Study the drawing (mm; zero at the part's minimum x, y, z) and answer. A direction names the side the tool comes from. Round coordinates to 2 decimals unless told otherwise and drop trailing zeros. Write each loop counter-clockwise with the first axis right and the second up, starting at its lowest first coordinate (ties: lowest second). Pieces come first, ordered by that corner, then holes. Notation, with made-up numbers: M 1,34 L 33,34 A23 cw 33,62 Z; hole C 45,-40 d10. An arc over 180 degrees is marked long. Write each question's results on one line, items separated by ' | '.
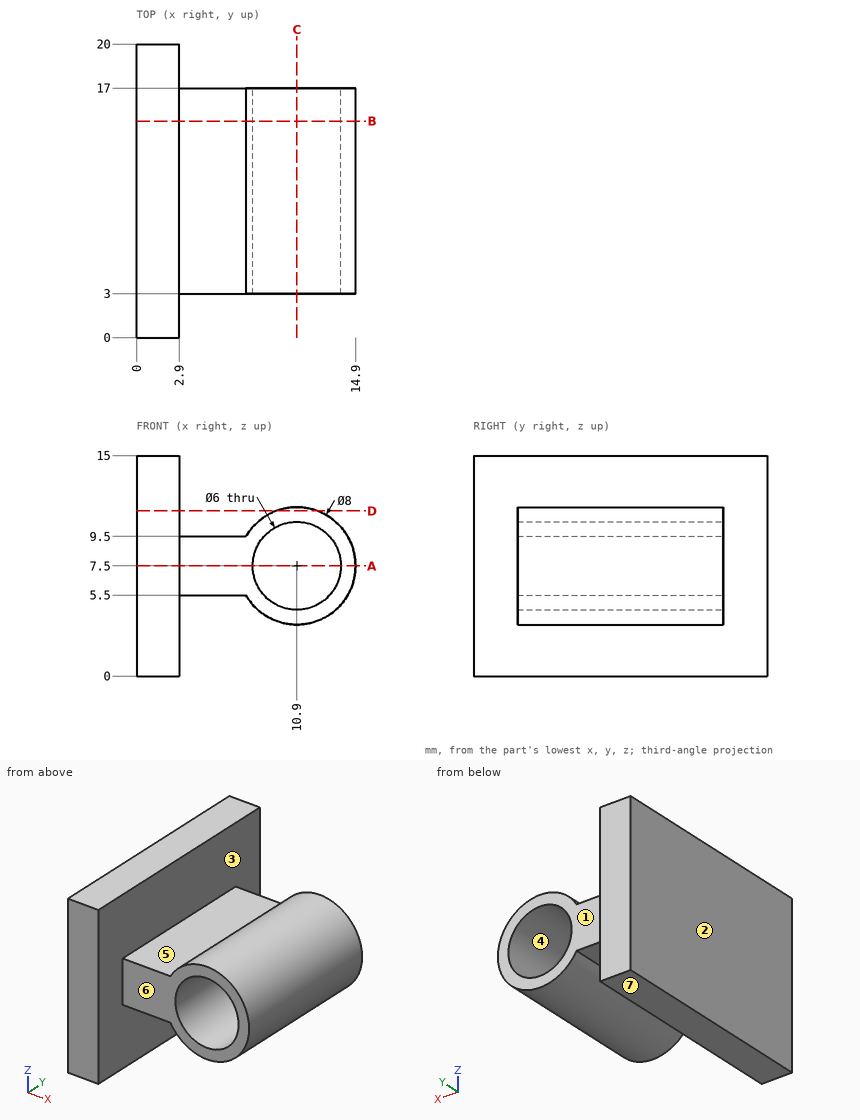
1) Find the intervals of material crossed by line 1 (Z direction, x = 10.9, y = 6.75); line 2 (X direction, y = 11.5, z = 7.5); line 3 (X direction, y = 15.75, z = 0.5), in increasing order.
Return value:
line 1: 3.5 to 4.5, 10.5 to 11.5 | line 2: 0 to 7.9, 13.9 to 14.9 | line 3: 0 to 2.9
2) Section D-D (z = 11.25) is taken. Determine the outline of the cut face in (x, y).
Return value:
outline: M 0,0 L 2.9,0 L 2.9,20 L 0,20 Z; M 9.51,3 L 12.29,3 L 12.29,17 L 9.51,17 Z
3) Section C-C (x = 10.9) is taken. Determine the outline of the cut face in (y, z), then the cut area to 3 significant figures.
Return value:
outline: M 3,3.5 L 17,3.5 L 17,4.5 L 3,4.5 Z; M 3,10.5 L 17,10.5 L 17,11.5 L 3,11.5 Z | area: 28.0 mm²
4) Section A-A (z = 7.5) is taken. Determine the outline of the cut face in (x, y).
Return value:
outline: M 0,0 L 2.9,0 L 2.9,3 L 7.9,3 L 7.9,17 L 2.9,17 L 2.9,20 L 0,20 Z; M 13.9,3 L 14.9,3 L 14.9,17 L 13.9,17 Z
5) The mould has two halves that part along X. Classify the marked faces 1, 2, 3 and 4: +X half, -X half, draft (parallel to the pull), parting line (faces both ways), or undercut.
Return value:
face 1: draft | face 2: -X half | face 3: undercut | face 4: undercut
6) Section B-B (y = 14.75) is taken. Determine the outline of the cut face in (x, z).
Return value:
outline: M 0,0 L 2.9,0 L 2.9,5.5 L 7.44,5.5 A4 ccw long 7.44,9.5 L 2.9,9.5 L 2.9,15 L 0,15 Z; hole C 10.9,7.5 d6
7) A tool of negligible diameter and unlimited length cuts with its end or side. For the marked faces 5, 6 and 7, from which of +Z, -Z, +X, -X, +Y, -Y can it reach the whole face along a straight path? Write none if from no direction.
Return value:
face 5: +Z, +Y, -Y | face 6: +Z, -Z, +X, -Y | face 7: -Z, +X, -X, +Y, -Y
8) Each of these flat-tipped pins is pushed along its axis until it touches: pin 1 (3 mm diameter, centred on x = 10, z = 4, fed in from -Y); pin 2 (4 mm diameter, centred on x = 8, z = 8.5, fed in from +Y); pin 3 (2.5 mm diameter, centred on x = 5, y = 12, fed in from -Z). Where does it stop, or does it pass through?
Return value:
pin 1: y = 3 | pin 2: y = 17 | pin 3: z = 5.5
